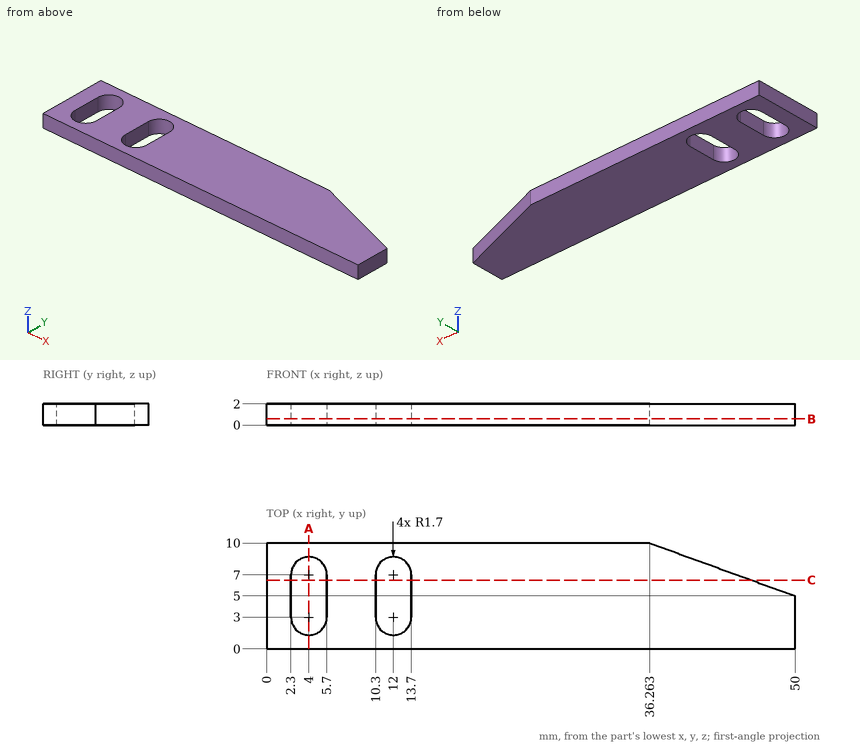
The figure shows three views and two pictorial views of one solid part (mm, origin at its lowest corner). Answer the questions. Round coordinates to 2 decimals unless told otherwise and drop trailing zeros. Write each loop counter-clockwise with the first axis right and the second up, starting at its lowest first coordinate (ties: lowest second). Pieces come first, ordered by that corner, then holes. Notation, with made-up numbers: (27, 37.5) -> (68, 37.5) arc R22 cw to (68, 66.5) -> close; hole circle Ø3 at (-24, -6). An arc over 180 degrees is marked (long way). Answer as a JSON object with one key per item and string values. Group by question number.
Q1. Section C-C (y = 6.5) is taken. Write down the section's boundary in (x, z).
Q2. Straight lines are drawn through the part: line 1 along X through (y, z) = (4, 1.65); line 2 along X through (y, z) = (1.5, 0.85); line 3 along Y through (x, z) = (46.5, 0.1) (1 decimal). For each, find the intervals that lie inside material, in ascending order.
Q3. Section B-B (z = 0.6) is taken. Write down the section's boundary in (x, y), plus the area to 3 significant figures.
Q4. Section A-A (x = 4) is taken. Write down the section's boundary in (y, z).
Check values:
{
 "1": {"outline": "(0, 0) -> (2.3, 0) -> (2.3, 2) -> (0, 2) -> close; (5.7, 0) -> (10.3, 0) -> (10.3, 2) -> (5.7, 2) -> close; (13.7, 0) -> (45.88, 0) -> (45.88, 2) -> (13.7, 2) -> close"},
 "2": {"line 1": "0 to 2.3, 5.7 to 10.3, 13.7 to 50", "line 2": "0 to 3.2, 4.8 to 11.2, 12.8 to 50", "line 3": "0 to 6.3"},
 "3": {"outline": "(0, 0) -> (50, 0) -> (50, 5) -> (36.26, 10) -> (0, 10) -> close; hole (2.3, 3) arc R1.7 ccw to (5.7, 3) -> (5.7, 7) arc R1.7 ccw to (2.3, 7) -> close; hole (10.3, 3) arc R1.7 ccw to (13.7, 3) -> (13.7, 7) arc R1.7 ccw to (10.3, 7) -> close", "area": "420 mm^2"},
 "4": {"outline": "(0, 0) -> (1.3, 0) -> (1.3, 2) -> (0, 2) -> close; (8.7, 0) -> (10, 0) -> (10, 2) -> (8.7, 2) -> close"}
}
